```python
from build123d import *

# Parameters (mm, degrees)
SZKIC1_R                    = 27.5
DODANIE_WYCI_GNI_CIE1_DEPTH = 30
SZKIC2_R                    = 40
DODANIE_WYCI_GNI_CIE2_DEPTH = 9.7
SZKIC3_W                    = 108.783825326
SZKIC3_H                    = 7.5
WYTNIJ_WYCI_GNI_CIE1_DEPTH  = 9.7
SZKIC5_W                    = 108.783825325
SZKIC5_H                    = 7.5
WYTNIJ_WYCI_GNI_CIE2_DEPTH  = 9.7
SZKIC6_R                    = 12.35
WYTNIJ_WYCI_GNI_CIE3_DEPTH  = 39.7
SZKIC7_R                    = 2.5
WYTNIJ_WYCI_GNI_CIE4_DEPTH  = 9.7


with BuildPart() as part:
    # Szkic1 → Dodanie-wyciągnięcie1 (new body)
    with BuildSketch(Plane.XY):
        Circle(SZKIC1_R)
    extrude(amount=DODANIE_WYCI_GNI_CIE1_DEPTH)

    # Szkic2 → Dodanie-wyciągnięcie2 (add)
    with BuildSketch(Plane.XY.offset(30)):
        Circle(SZKIC2_R)
    extrude(amount=DODANIE_WYCI_GNI_CIE2_DEPTH)

    # Szkic3 → Wytnij-wyciągnięcie1 (cut)
    with BuildSketch(Plane.XY.offset(39.7)):
        with Locations((-0.621798063, 36.25)):
            Rectangle(SZKIC3_W, SZKIC3_H)
    extrude(amount=-WYTNIJ_WYCI_GNI_CIE1_DEPTH, mode=Mode.SUBTRACT)

    # Szkic5 → Wytnij-wyciągnięcie2 (cut)
    with BuildSketch(Plane.XY.offset(39.7)):
        with Locations((-3.409138593, -36.25)):
            Rectangle(SZKIC5_W, SZKIC5_H)
    extrude(amount=-WYTNIJ_WYCI_GNI_CIE2_DEPTH, mode=Mode.SUBTRACT)

    # Szkic6 → Wytnij-wyciągnięcie3 (cut)
    with BuildSketch(Plane.XY):
        Circle(SZKIC6_R)
    extrude(amount=WYTNIJ_WYCI_GNI_CIE3_DEPTH, mode=Mode.SUBTRACT)

    # Szkic7 → Wytnij-wyciągnięcie4 (cut)
    with BuildSketch(Plane.XY.offset(39.7)):
        with Locations((-24, 24)):
            Circle(SZKIC7_R)
        with Locations((24, 24)):
            Circle(SZKIC7_R)
        with Locations((-24, -24)):
            Circle(SZKIC7_R)
        with Locations((24, -24)):
            Circle(SZKIC7_R)
    extrude(amount=-WYTNIJ_WYCI_GNI_CIE4_DEPTH, mode=Mode.SUBTRACT)


solid = part.part
```
Geometry check sheet. Reference: the model listing, model coordinates, mm. A direction names the side the tool comes from. Give positions to 0.01 mm unless a question says otherwise; leave off trailing zeros. Order: outer loops, then holes, each group sorted by start corner. A loop starts at its lowest first (then second) coordinate and runs counter-clockwise, first axis right, second up. Notation, with made-up numbers: (83.5, 89) -> (133.5, 89) arc R24 cw to (133.5, 116) -> close; hole circle Ø7 at (-27, 18). An arc over 180 degrees is marked (long way). Write each question's results on one line, items separated by ' | '. Start each with the question number.
(1) Sectioned sample at B-B (z = 32). Enter the section's corners in (x, y), plus the area to 3 significant figures.
(2) Gauge pin test, flat ends, axial feed: P1, Ø4, axis at x = 26, z = 21.5, coming from the -Y side; P2, Ø4, axis at x = -26, y = -20, coming from the -Z side; P3, Ø5, axis at y = -23, z = 32.5, coming from the +X side. Record the tip position at first contact, or that the pin passes through.
(3) Access from +Z, -Z, +X, -X, +Y, -Y to the whole of each face (thin tool, end or side, straight path). Record for faces 5 (the face through (39.996, -0.531, 34.782)), 6 (the face through (-5.961, -26.846, 14.79)).
(4) Sectioned sample at C-C (y = 0). Enter the section's corners in (x, z).
(5) Sectioned sample at D-D (z = 9.5). Enter the section's corners in (x, y).
(6) Scan lines: line 1 (Y direction, x = 24, z = 36.75); line 2 (Y direction, x = 22, z = 34.5); line 3 (Z direction, x = -36, y = -4). Record each from-to range of solid material in increasing order.
(7) Sectioned sample at A-A (x = 0). Enter the section's corners in (y, z), plus the area to 3 significant figures.
(8) Mould release check, pull along Y, two halves, no side actions. Record for faces 1 (the face through (-25.84, 25.69, 34.92)), 2 (the face through (-39.996, 0.531, 34.782)), 3 (the face through (6, -12, 0)), 4 (the face through (0, -32.5, 35)): pulls with the +Y half, pulls with the -Y half, needs draft (parallel to the pull), parting line crosses it, or undercut.
Answer below:
1) outline: (-23.32, -32.5) -> (23.32, -32.5) arc R40 ccw to (23.32, 32.5) -> (-23.32, 32.5) arc R40 ccw to start; hole circle Ø5 at (-24, -24); hole circle Ø5 at (-24, 24); hole circle Ø24.7 at (0, 0); hole circle Ø5 at (24, -24); hole circle Ø5 at (24, 24) | area: 3,990 mm2
2) P1: y = -13.43 | P2: z = 30 | P3: x = 34.35
3) face 5: +Z, -Z, +X | face 6: -Z
4) outline: (-40, 30) -> (-27.5, 30) -> (-27.5, 0) -> (-12.35, 0) -> (-12.35, 39.7) -> (-40, 39.7) -> close; (12.35, 0) -> (27.5, 0) -> (27.5, 30) -> (40, 30) -> (40, 39.7) -> (12.35, 39.7) -> close
5) outline: circle Ø55 at (0, 0); hole circle Ø24.7 at (0, 0)
6) line 1: -32 to -26.5, -21.5 to 21.5, 26.5 to 32 | line 2: -32.5 to -25.5, -22.5 to 22.5, 25.5 to 32.5 | line 3: 30 to 39.7
7) outline: (-32.5, 30) -> (-27.5, 30) -> (-27.5, 0) -> (-12.35, 0) -> (-12.35, 39.7) -> (-32.5, 39.7) -> close; (12.35, 0) -> (27.5, 0) -> (27.5, 30) -> (32.5, 30) -> (32.5, 39.7) -> (12.35, 39.7) -> close | area: 1,300 mm2
8) face 1: undercut | face 2: parting line crosses it | face 3: needs draft | face 4: pulls with the -Y half
